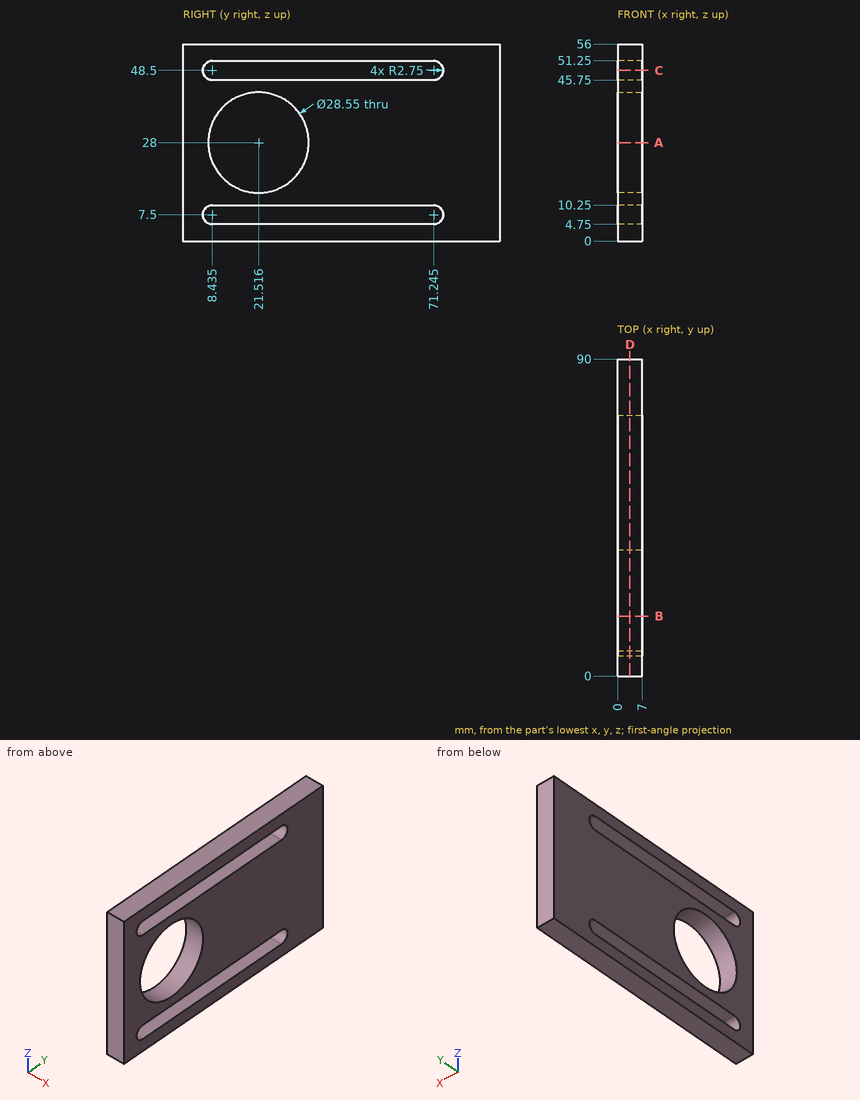
Drawing for the job (mm, zero at the part's lowest x, y, z). Give positions to 0.01 mm unless a question says otherwise; leave off trailing zeros. Order: outer loops, then holes, each group sorted by start corner. A loop starts at its lowest first (then second) coordinate and runs counter-clockwise, first axis right, second up. Notation, with made-up numbers: M 82.5,83.5 L 91.5,83.5 A22 cw 91.5,122.5 Z; hole C -17,-8 d5. An arc over 180 degrees is marked long. Write item = value, one per line. Start each with the question number.
(1) Slice it at B-B on y = 17. Write the cut outline in (x, z).
(2) Slice it at D-D on x = 3.5. State how many separate pieces and enclosed holes the cut face has, plus the area to 3 significant figures.
(3) Slice it at C-C on z = 48.5. Write the cut outline in (x, y) (1 decimal), plus the area to 3 significant figures.
(4) Probe L1, parallel to Z at x = 1, y = 56; L2, parallel to Y at x = 4.75, z = 28; L3, parallel to Z at x = 1, y = 22.5. List the from-to ranges inside material, lowest first. Write a range as [from, to].
(5) Slice it at A-A on z = 28. Write the cut outline in (x, y), plus the area to 3 significant figures.
Responses:
q1.outline = M 0,0 L 7,0 L 7,4.75 L 0,4.75 Z; M 0,10.25 L 7,10.25 L 7,14.46 L 0,14.46 Z; M 0,41.54 L 7,41.54 L 7,45.75 L 0,45.75 Z; M 0,51.25 L 7,51.25 L 7,56 L 0,56 Z
q2.separate_pieces = 1
q2.enclosed_holes = 3
q2.area = 3,660 mm2
q3.outline = M 0,0 L 7,0 L 7,5.7 L 0,5.7 Z; M 0,74 L 7,74 L 7,90 L 0,90 Z
q3.area = 152 mm2
q4.L1 = [0, 4.75], [10.25, 45.75], [51.25, 56]
q4.L2 = [0, 7.24], [35.79, 90]
q4.L3 = [0, 4.75], [10.25, 13.76], [42.24, 45.75], [51.25, 56]
q5.outline = M 0,0 L 7,0 L 7,7.24 L 0,7.24 Z; M 0,35.79 L 7,35.79 L 7,90 L 0,90 Z
q5.area = 430 mm2
